from build123d import *

# Parameters (mm, degrees)
SKETCH1_W                                  = 70
SKETCH1_H                                  = 15
BOSS_EXTRUDE1_DEPTH                        = 3
SKETCH2_W                                  = 7
SKETCH2_H                                  = 15
BOSS_EXTRUDE2_DEPTH                        = 10
SKETCH5_R                                  = 4.5
CUT_EXTRUDE1_DEPTH                         = 72.590851371
SKETCH6_R                                  = 6.1
CUT_EXTRUDE4_DEPTH                         = 2.1
BOSS_EXTRUDE3_DEPTH                        = 13
SKETCH8_R                                  = 2
CUT_EXTRUDE5_DEPTH                         = 40.534794802
SKETCH9_R                                  = 1.75
CUT_EXTRUDE6_DEPTH                         = 39.65229618
MIRROR1_AT_THE_SECOND_PLANE_COPY_1_SKETC_R = 6.1
MIRROR1_AT_THE_SECOND_PLANE_COPY_1_DEPTH   = 2.1
MIRROR1_AT_THE_SECOND_PLANE_COPY_2_DEPTH   = 13
MIRROR1_AT_THE_SECOND_PLANE_COPY_3_SKETC_R = 2
MIRROR1_AT_THE_SECOND_PLANE_COPY_3_DEPTH   = 40.534794802
MIRROR1_AT_THE_SECOND_PLANE_COPY_4_SKETC_R = 1.75
MIRROR1_AT_THE_SECOND_PLANE_COPY_4_DEPTH   = 39.65229618
FILLET1_R                                  = 6
SKETCH10_W                                 = 56
SKETCH10_H                                 = 23
BOSS_EXTRUDE4_DEPTH                        = 15
FILLET2_R                                  = 4
SKETCH11_R                                 = 13
CUT_EXTRUDE7_DEPTH                         = 66.627738058
SKETCH12_W                                 = 8
SKETCH12_H                                 = 9.596439054
BOSS_EXTRUDE5_DEPTH                        = 7
BOSS_EXTRUDE5_DIRECTION_2_REACH            = 46.657
FILLET3_R                                  = 4
SKETCH13_R                                 = 1.75
CUT_EXTRUDE8_DEPTH                         = 46.948340586
SKETCH14_W                                 = 7
SKETCH14_H                                 = 26
BOSS_EXTRUDE6_DEPTH                        = 5
SKETCH15_W                                 = 7
SKETCH15_H                                 = 26
BOSS_EXTRUDE7_DEPTH                        = 14
FILLET5_R                                  = 4
SKETCH16_R                                 = 5.5
CUT_EXTRUDE9_DEPTH                         = 75.854859562
FILLET3_OF_MIRROR2_R                       = 4
FILLET5_OF_MIRROR2_R                       = 4
SKETCH17_R                                 = 1.25
CUT_EXTRUDE10_DEPTH                        = 75.854859562
CUT_EXTRUDE14_DEPTH                        = 31
CUT_EXTRUDE14_DEPTH_BACK                   = 31
SKETCH18_R                                 = 12.95


with BuildPart() as part:
    # Sketch1 → Boss-Extrude1 (new body)
    with BuildSketch(Plane.XY):
        Rectangle(SKETCH1_W, SKETCH1_H)
    extrude(amount=BOSS_EXTRUDE1_DEPTH)

    # Sketch2 → Boss-Extrude2 (add)
    with BuildSketch(Plane.XY.offset(3)):
        with Locations((-31.5, 0)):
            Rectangle(SKETCH2_W, SKETCH2_H)
        with Locations((31.5, 0)):
            Rectangle(SKETCH2_W, SKETCH2_H)
    extrude(amount=BOSS_EXTRUDE2_DEPTH)

    # Sketch5 → Cut-Extrude1 (cut, through all)
    with BuildSketch(Plane(origin=(35, 0, 0), x_dir=(0, 0, -1), z_dir=(1, 0, 0))):
        with Locations((-13, 0)):
            Circle(SKETCH5_R)
    extrude(amount=-CUT_EXTRUDE1_DEPTH, mode=Mode.SUBTRACT)

    # Sketch6 → Cut-Extrude4 (cut, symmetric)
    with BuildSketch(Plane(origin=(31.5, 0, 0), x_dir=(0, 0, -1), z_dir=(1, 0, 0))):
        with Locations((-13, 0)):
            Circle(SKETCH6_R)
    cut_extrude4 = extrude(amount=CUT_EXTRUDE4_DEPTH, both=True, mode=Mode.SUBTRACT)

    # Sketch7 → Boss-Extrude3 (add)
    with BuildSketch(Plane.XY):
        Polygon((28, 8.1), (28, 13), (35, 13), (35, 8.1), (35, 4.5), (33.6, 4.5), (33.6, 6.1), (29.4, 6.1), (29.4, 4.5), (28, 4.5), align=None)
    boss_extrude3 = extrude(amount=BOSS_EXTRUDE3_DEPTH)

    # Sketch8 → Cut-Extrude5 (cut, symmetric)
    with BuildSketch(Plane.XY.offset(13)):
        with Locations((31.5, 10)):
            Circle(SKETCH8_R)
    cut_extrude5 = extrude(amount=CUT_EXTRUDE5_DEPTH, both=True, mode=Mode.SUBTRACT)

    # Sketch9 → Cut-Extrude6 (cut, through all)
    with BuildSketch(Plane.XY.offset(3)):
        with Locations((-10, -4)):
            Circle(SKETCH9_R)
    cut_extrude6 = extrude(amount=-CUT_EXTRUDE6_DEPTH, mode=Mode.SUBTRACT)

    # Mirror1: Cut-Extrude4, Boss-Extrude3, Cut-Extrude5, Cut-Extrude6 across plane
    add(cut_extrude4.mirror(Plane(origin=(0, 0, 0), x_dir=(0, 0, 1), z_dir=(1, 0, 0))), mode=Mode.SUBTRACT)
    add(boss_extrude3.mirror(Plane(origin=(0, 0, 0), x_dir=(0, 0, 1), z_dir=(1, 0, 0))))
    add(cut_extrude5.mirror(Plane(origin=(0, 0, 0), x_dir=(0, 0, 1), z_dir=(1, 0, 0))), mode=Mode.SUBTRACT)
    add(cut_extrude6.mirror(Plane(origin=(0, 0, 0), x_dir=(0, 0, 1), z_dir=(1, 0, 0))), mode=Mode.SUBTRACT)

    # Mirror1 at the second plane: Cut-Extrude4, Boss-Extrude3, Cut-Extrude5, Cut-Extrude6 across plane
    add(cut_extrude4.mirror(Plane.ZX), mode=Mode.SUBTRACT)
    add(boss_extrude3.mirror(Plane.ZX))
    add(cut_extrude5.mirror(Plane.ZX), mode=Mode.SUBTRACT)
    add(cut_extrude6.mirror(Plane.ZX), mode=Mode.SUBTRACT)

    # Mirror1 at the second plane copy 1 sketc → Mirror1 at the second plane copy 1 (cut, symmetric)
    with BuildSketch(Plane(origin=(-31.5, 0, 0), x_dir=(0, 0, -1), z_dir=(-1, 0, 0))):
        with Locations((-13, 0)):
            Circle(MIRROR1_AT_THE_SECOND_PLANE_COPY_1_SKETC_R)
    extrude(amount=MIRROR1_AT_THE_SECOND_PLANE_COPY_1_DEPTH, both=True, mode=Mode.SUBTRACT)

    # Mirror1 at the second plane copy 2 sketc → Mirror1 at the second plane copy 2 (add)
    with BuildSketch(Plane(origin=(0, 0, 0), x_dir=(-1, 0, 0), z_dir=(0, 0, 1))):
        Polygon((28, 8.1), (28, 13), (35, 13), (35, 8.1), (35, 4.5), (33.6, 4.5), (33.6, 6.1), (29.4, 6.1), (29.4, 4.5), (28, 4.5), align=None)
    extrude(amount=MIRROR1_AT_THE_SECOND_PLANE_COPY_2_DEPTH)

    # Mirror1 at the second plane copy 3 sketc → Mirror1 at the second plane copy 3 (cut, symmetric)
    with BuildSketch(Plane(origin=(0, 0, 13), x_dir=(-1, 0, 0), z_dir=(0, 0, 1))):
        with Locations((31.5, 10)):
            Circle(MIRROR1_AT_THE_SECOND_PLANE_COPY_3_SKETC_R)
    extrude(amount=MIRROR1_AT_THE_SECOND_PLANE_COPY_3_DEPTH, both=True, mode=Mode.SUBTRACT)

    # Mirror1 at the second plane copy 4 sketc → Mirror1 at the second plane copy 4 (cut, through all)
    with BuildSketch(Plane(origin=(0, 0, 3), x_dir=(-1, 0, 0), z_dir=(0, 0, 1))):
        with Locations((-10, -4)):
            Circle(MIRROR1_AT_THE_SECOND_PLANE_COPY_4_SKETC_R)
    extrude(amount=-MIRROR1_AT_THE_SECOND_PLANE_COPY_4_DEPTH, mode=Mode.SUBTRACT)

    # Fillet1
    fillet1_edges = [part.edges().sort_by_distance(p)[0] for p in [
        (-28, 0, 3),
        (28, 0, 3),
    ]]
    fillet(fillet1_edges, radius=FILLET1_R)

    # Sketch10 → Boss-Extrude4 (add)
    with BuildSketch(Plane(origin=(0, 0, 3), x_dir=(-1, 0, 0), z_dir=(0, 0, -1))):
        Rectangle(SKETCH10_W, SKETCH10_H)
    extrude(amount=BOSS_EXTRUDE4_DEPTH)

    # Fillet2
    # the kernel refuses this fillet: 4 mm, written as the material it takes off along each edge
    with BuildSketch(Plane(origin=(-28, 11.5, 3), x_dir=(0, 0, -1), z_dir=(1, 0, 0)), Plane(origin=(28, -11.5, 3), x_dir=(0, 0, -1), z_dir=(-1, 0, 0))) as fillet2_piece_1:
        with BuildLine():
            CenterArc((FILLET2_R, -FILLET2_R), FILLET2_R, 90, 90)
            Line((0, -FILLET2_R), (0, 0))
            Line((0, 0), (FILLET2_R, 0))
        make_face()
    extrude(amount=56, mode=Mode.SUBTRACT)

    # Sketch11 → Cut-Extrude7 (cut, through all)
    with BuildSketch(Plane(origin=(28, 0, 0), x_dir=(0, 0, -1), z_dir=(1, 0, 0))):
        with Locations((13, 0)):
            Circle(SKETCH11_R)
    extrude(amount=-CUT_EXTRUDE7_DEPTH, mode=Mode.SUBTRACT)

    # Sketch12 → Boss-Extrude5 (add)
    with BuildSketch(Plane.XZ.offset(11.5)):
        with Locations((-9, -2.139602647)):
            Rectangle(SKETCH12_W, SKETCH12_H)
    boss_extrude5 = extrude(amount=BOSS_EXTRUDE5_DEPTH)

    # Sketch12 → Boss-Extrude5 direction 2 (add, up to next)
    with BuildSketch(Plane.XZ.offset(11.5), mode=Mode.PRIVATE) as boss_extrude5_direction_2_sk1:
        with Locations((-9, -2.139602647)):
            Rectangle(SKETCH12_W, SKETCH12_H)
    boss_extrude5_direction_2_tool1 = extrude(boss_extrude5_direction_2_sk1.sketch, amount=-BOSS_EXTRUDE5_DIRECTION_2_REACH, mode=Mode.PRIVATE) - part.part
    boss_extrude5_direction_2 = boss_extrude5_direction_2_tool1.solids().sort_by_distance((-9, -11.5, -2.139603))[0]
    add(boss_extrude5_direction_2)

    # Fillet3
    fillet3_edges = [part.edges().sort_by_distance(p)[0] for p in [
        (-9, -18.5, 2.65861688),
        (-9, -18.5, -6.937822174),
    ]]
    fillet(fillet3_edges, radius=FILLET3_R)

    # Sketch13 → Cut-Extrude8 (cut, through all)
    with BuildSketch(Plane(origin=(-5, 0, 0), x_dir=(0, 0, -1), z_dir=(1, 0, 0))):
        with Locations((2.108513734, -15)):
            Circle(SKETCH13_R)
    cut_extrude8 = extrude(amount=-CUT_EXTRUDE8_DEPTH, mode=Mode.SUBTRACT)

    # Sketch14 → Boss-Extrude6 (add)
    with BuildSketch(Plane(origin=(0, 0, 0), x_dir=(-1, 0, 0), z_dir=(0, 0, -1))):
        with Locations((31.5, 0)):
            Rectangle(SKETCH14_W, SKETCH14_H)
    boss_extrude6 = extrude(amount=BOSS_EXTRUDE6_DEPTH)

    # Sketch15 → Boss-Extrude7 (add)
    with BuildSketch(Plane(origin=(0, 0, -5), x_dir=(-1, 0, 0), z_dir=(0, 0, -1))):
        with Locations((31.5, 0)):
            Rectangle(SKETCH15_W, SKETCH15_H)
    boss_extrude7 = extrude(amount=BOSS_EXTRUDE7_DEPTH)

    # Fillet5
    fillet5_edges = [part.edges().sort_by_distance(p)[0] for p in [
        (-31.5, 13, -19),
        (-31.5, -13, -19),
    ]]
    fillet(fillet5_edges, radius=FILLET5_R)

    # Sketch16 → Cut-Extrude9 (cut, through all)
    with BuildSketch(Plane.ZY.offset(35)):
        with Locations((-10, 0)):
            Circle(SKETCH16_R)
    cut_extrude9 = extrude(amount=-CUT_EXTRUDE9_DEPTH, mode=Mode.SUBTRACT)

    # Mirror2: Boss-Extrude5, Boss-Extrude5 direction 2, Cut-Extrude8, Boss-Extrude6, Boss-Extrude7, Cut-Extrude9 across plane
    add(boss_extrude5.mirror(Plane(origin=(0, 0, 0), x_dir=(0, 0, 1), z_dir=(1, 0, 0))))
    add(boss_extrude5_direction_2.mirror(Plane(origin=(0, 0, 0), x_dir=(0, 0, 1), z_dir=(1, 0, 0))))
    add(cut_extrude8.mirror(Plane(origin=(0, 0, 0), x_dir=(0, 0, 1), z_dir=(1, 0, 0))), mode=Mode.SUBTRACT)
    add(boss_extrude6.mirror(Plane(origin=(0, 0, 0), x_dir=(0, 0, 1), z_dir=(1, 0, 0))))
    add(boss_extrude7.mirror(Plane(origin=(0, 0, 0), x_dir=(0, 0, 1), z_dir=(1, 0, 0))))
    add(cut_extrude9.mirror(Plane(origin=(0, 0, 0), x_dir=(0, 0, 1), z_dir=(1, 0, 0))), mode=Mode.SUBTRACT)

    # Fillet3 of Mirror2
    fillet3_of_mirror2_edges = [part.edges().sort_by_distance(p)[0] for p in [
        (9, -18.5, 2.65861688),
        (9, -18.5, -6.937822174),
    ]]
    fillet(fillet3_of_mirror2_edges, radius=FILLET3_OF_MIRROR2_R)

    # Fillet5 of Mirror2
    fillet5_of_mirror2_edges = [part.edges().sort_by_distance(p)[0] for p in [
        (31.5, 13, -19),
        (31.5, -13, -19),
    ]]
    fillet(fillet5_of_mirror2_edges, radius=FILLET5_OF_MIRROR2_R)

    # Sketch17 → Cut-Extrude10 (cut, through all)
    with BuildSketch(Plane.ZY.offset(35)):
        with Locations((-13, 9.5)):
            Circle(SKETCH17_R)
        with Locations((-13, -9.5)):
            Circle(SKETCH17_R)
    extrude(amount=-CUT_EXTRUDE10_DEPTH, mode=Mode.SUBTRACT)

    # Sketch18 → Cut-Extrude14 (cut, two sides: drawn at the far end of the back side and taken through both)
    with BuildSketch(Plane(origin=(0, 0, 0), x_dir=(0, 0, -1), z_dir=(1, 0, 0)).offset(-CUT_EXTRUDE14_DEPTH_BACK)):
        with Locations((13, 0)):
            Circle(SKETCH18_R)
    extrude(amount=CUT_EXTRUDE14_DEPTH + CUT_EXTRUDE14_DEPTH_BACK, mode=Mode.SUBTRACT)


solid = part.part
Input: part model. Units: mm. Frame: model coordinates. A direction names the side the tool comes from. Give positions to 0.01 mm unless a question says otherwise; leave off trailing zeros. Loops run counter-clockwise (first coordinate to the right, second up) from the corner with the lowest first, then second, coordinate; pieces in that order, holes last. Notation, with made-up numbers: M 49.25,15 L 58.25,15 A19 cw 58.25,36 Z; hole C 85.25,20.5 d2. An arc over 180 degrees is marked long. Use CSV: the item, a comma, the result in double quotes.
(1) Pull-direction query (Y, two-part tool) for faces 1 (the face through (31, 10, 0)), 2 (the face through (-5, -13, -2)), 3 (the face through (-8.944, -17.297, -5.797)); classes: pulls with the +Y half, pulls with the -Y half, needs draft (parallel to the pull), parting line crosses it, or undercut.
Outcome:
face 1,"undercut"
face 2,"needs draft"
face 3,"pulls with the -Y half"
(2) Pin query (flat end, axial travel): P1, Ø4.5, axis at x = -7, y = -11.5, coming from the +Z side; P2, Ø1, axis at x = -21, y = -2, coming from the +Z side; P3, Ø3, axis at x = 24, y = -5.5, coming from the +Z side. Return the tip coordinate at first contact, or that it passes through.
Outcome:
P1,"stops at z = 2.66"
P2,"stops at z = 3"
P3,"stops at z = 4.13"
(3) Section B-B, the plane x = 18.5. Return loops of the section in (y, z).
Outcome:
outline,"M -11.5,-6.94 A13 cw 11.5,-6.94 L 11.5,-1 A4 ccw 7.5,3 L -7.5,3 A4 ccw -11.5,-1 Z"
(4) Set-up query: faces 4 (the face through (33.408, 10.601, 6.591)), 5 (the face through (-29.521, 0.348, -0.055)), 6 (the face through (9, -13, -6.938)), 7 (the face through (0, -11.5, -4)), 8 (the face through (32.3, -7.9, 13)). Return all of +Z, -Z, +X, -X, +Y, -Y with unobstructed straight access to the full face (end or side cutting, diameter ignored); none if empty.
Outcome:
face 4,"+Z"
face 5,"none"
face 6,"-Z, +Y, -Y"
face 7,"+Z, -Z, -Y"
face 8,"+Z, +X, -X, +Y, -Y"
(5) Section A-A, the plane y = 0. Count the separate pieces of the cut face and the enclosed holes in it, plus the area to 3 significant figures.
Outcome:
separate pieces,"3"
enclosed holes,"0"
area,"353 mm²"
(6) Material intervals for L1, parallel to X at y = -14, z = 0; L2, parallel to X at y = 12, z = -5; L3, parallel to X at y = 9, z = 6.5, sorted ascending. Write a range as [from, to].
Outcome:
L1,"x = [-13, -5], [5, 13]"
L2,"x = [-35, -28], [28, 35]"
L3,"x = [-35, -33.23], [-29.77, -28], [28, 29.77], [33.23, 35]"
